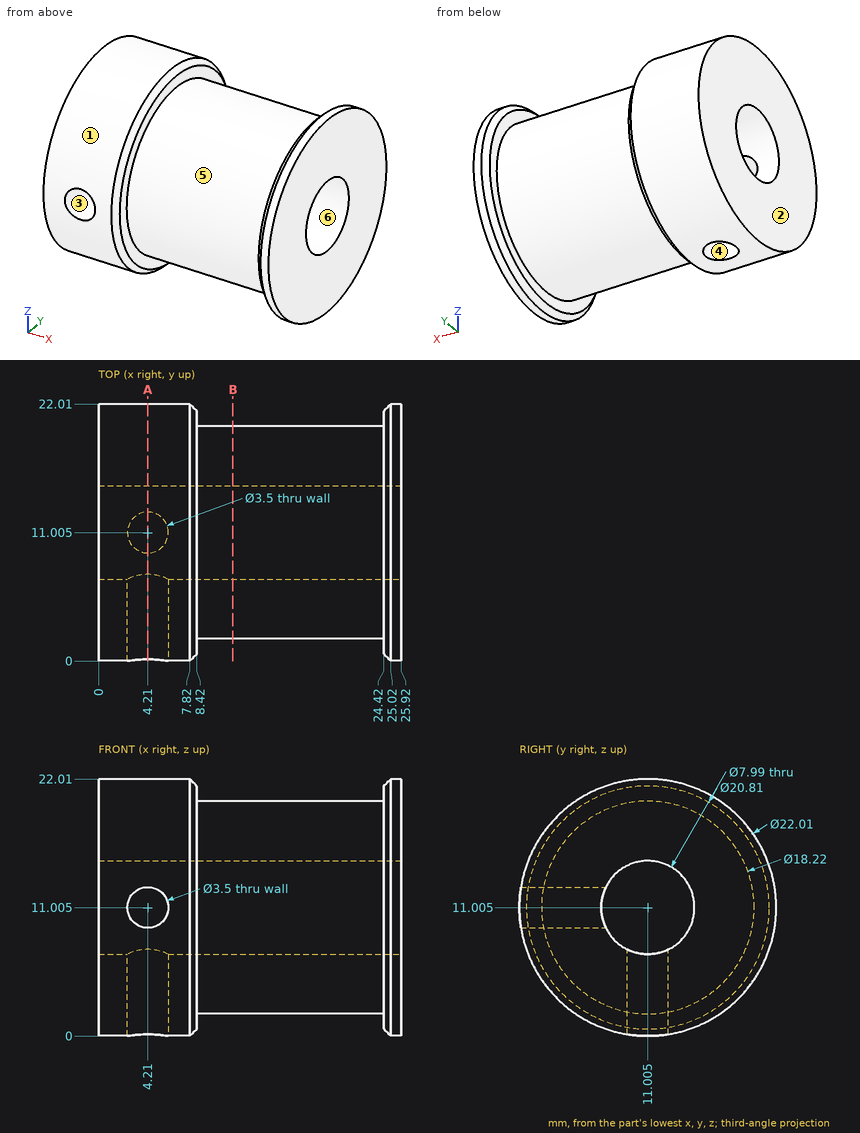
Source: three-view drawing plus pictorial views. Frame: mm from the lowest corner of the part. A direction names the side the tool comes from. Coordinates: 2 decimals unless noted, no trailing zeros. Loops run counter-clockwise (first coordinate to the right, second up) from the corner with the lowest first, then second, coordinate; pieces in that order, holes last. Notation, with made-up numbers: (-19, 66.25) - (24, 66.25) arc R15 ccw to (24, 93.25) - close; hole circle Ø3 at (55.25, 32.5). An arc over 180 degrees is marked (long way). Answer in a Markdown table with one row per item. Add a question column.
Item 1: Section query A-A on x = 4.21. Return the cut outline in (y, z) (3 decimals), then the cut area to 3 significant figures.
Item 2: Mould query, pull axis Z, two halves, no side actions, for the marked faces 1, 2 and 3. Classes: released by +Z, released by -Z, zero draft, split by the parting line, or undercut.
Item 3: Access query for the marked faces 4, 5 and 6. Directions: +Z, -Z, +X, -X, +Y, -Y. A direction counts if a zero-diameter tool reaches every point of the face in a straight line with its end or side. Return the directions, or none.
Item 4: Section query B-B on x = 11.5. Return the cut outline in (y, z) (3 decimals).
Item 5: Line query: line 1 along X through (y, z) = (19.25, 16.5); line 2 along Z through (x, y) = (2.25, 9.5); line 3 along Z through (x, y) = (21.75, 13.5). Output: solid intervals per line, ascending. Write a range as [from, to].
Item 6: Contact query for flat-ended pins moving along their axis: P1, Ø3, axis at x = 13.5, z = 11, coming from the +Y side (3 decimals); P2, Ø1.5, axis at x = 10, z = 6.5, coming from the +Y side; P3, Ø8, axis at x = 21, y = 15.5, coming from the -Z side. Output: stop coordinate, or through.
Recorded:
| question | item | result |
|---|---|---|
| 1 | outline | (0.14, 9.255) arc R11.005 ccw to (9.255, 0.14) - (9.255, 7.414) arc R3.995 cw to (7.414, 9.255) - close; (0.14, 12.755) - (7.414, 12.755) arc R3.995 cw (long way) to (12.755, 7.414) - (12.755, 0.14) arc R11.005 ccw (long way) to start |
| 1 | area | 281 mm^2 |
| 2 | face 1 | split by the parting line |
| 2 | face 2 | zero draft |
| 2 | face 3 | undercut |
| 3 | face 4 | -Z |
| 3 | face 5 | none |
| 3 | face 6 | +X, -X |
| 4 | outline | circle Ø18.22 at (11.005, 11.005); hole circle Ø7.99 at (11.005, 11.005) |
| 5 | line 1 | [0, 8.42], [24.42, 25.92] |
| 5 | line 2 | [0.1, 7.3], [14.71, 21.91] |
| 5 | line 3 | [2.24, 7.88], [14.13, 19.77] |
| 6 | P1 | y = 20.115 |
| 6 | P2 | y = 19.31 |
| 6 | P3 | z = 0.72 |
